```python
from build123d import *

# Parameters (mm, degrees)
BOSS_EXTRUDE1_DEPTH = 1.5
SKETCH3_R           = 7.5
SKETCH3_R_2         = 1.5
SKETCH3_W           = 12
SKETCH3_H           = 23
SKETCH3_W_2         = 5.25
SKETCH3_H_2         = 1.5
CUT_EXTRUDE1_DEPTH  = 66.639165138


with BuildPart() as part:
    # Sketch2 → Boss-Extrude1 (new body)
    with BuildSketch(Plane(origin=(0, 0, 0), x_dir=(1, 0, 0), z_dir=(0, 1, 0))):
        with BuildLine():
            Line((-26.339134382, 42.5), (26.339134382, 42.5))
            ThreePointArc((26.339134382, 42.5), (50, 0), (26.339134382, -42.5))
            Line((26.339134382, -42.5), (-26.339134382, -42.5))
            ThreePointArc((-26.339134382, -42.5), (-50, 0), (-26.339134382, 42.5))
        make_face()
    extrude(amount=BOSS_EXTRUDE1_DEPTH)

    # Sketch3 → Cut-Extrude1 (cut, through all)
    with BuildSketch(Plane(origin=(0, 1.5, 0), x_dir=(1, 0, 0), z_dir=(0, 1, 0))):
        with Locations(Location((0, 0, 0), (0, 0, 270))):
            Circle(SKETCH3_R)
        with Locations(Location((-47, 0, 0), (0, 0, 270))):
            Circle(SKETCH3_R_2)
        with Locations(Location((-33.466401061, 33, 0), (0, 0, 270))):
            Circle(SKETCH3_R_2)
        with Locations(Location((-12.966401061, 33, 0), (0, 0, 270))):
            Circle(SKETCH3_R_2)
        with Locations(Location((-40, 0, 0), (0, 0, 270))):
            Circle(SKETCH3_R_2)
        with Locations(Location((-12.966401061, -33, 0), (0, 0, 90))):
            Circle(SKETCH3_R_2)
        with Locations(Location((-33.466401061, -33, 0), (0, 0, 90))):
            Circle(SKETCH3_R_2)
        with Locations(Location((33.466401061, 33, 0), (0, 0, 90))):
            Circle(SKETCH3_R_2)
        with Locations(Location((12.966401061, 33, 0), (0, 0, 90))):
            Circle(SKETCH3_R_2)
        with Locations(Location((12.966401061, -33, 0), (0, 0, 270))):
            Circle(SKETCH3_R_2)
        with Locations(Location((33.466401061, -33, 0), (0, 0, 270))):
            Circle(SKETCH3_R_2)
        with Locations(Location((40, 0, 0), (0, 0, 90))):
            Circle(SKETCH3_R_2)
        with Locations(Location((47, 0, 0), (0, 0, 90))):
            Circle(SKETCH3_R_2)
        with Locations((-31, -5)):
            Rectangle(SKETCH3_W, SKETCH3_H)
        with Locations((0, -22.5)):
            Rectangle(SKETCH3_W_2, SKETCH3_H_2)
        with Locations((-9.95, 22.5)):
            Rectangle(SKETCH3_W_2, SKETCH3_H_2)
        with Locations((0, 22.5)):
            Rectangle(SKETCH3_W_2, SKETCH3_H_2)
        with Locations((-9.95, -22.5)):
            Rectangle(SKETCH3_W_2, SKETCH3_H_2)
    extrude(amount=-CUT_EXTRUDE1_DEPTH, mode=Mode.SUBTRACT)


solid = part.part
```
Verification items for the finished model (mm, model axes). Coordinates: 2 decimals unless noted, no trailing zeros. Loops run counter-clockwise (first coordinate to the right, second up) from the corner with the lowest first, then second, coordinate; pieces in that order, holes last. Notation, with made-up numbers: (-35, 82.5) -> (3, 82.5) arc R32 cw to (3, 118.5) -> close; hole circle Ø5 at (68, 7.5). An arc over 180 degrees is marked (long way). Answer in a Markdown table with one row per item.
1) Section check B-B (z = 0). Record the cut outline in (x, y).
The answers:
| item | result |
|---|---|
| outline | (-50, 0) -> (-48.5, 0) -> (-48.5, 1.5) -> (-50, 1.5) -> close; (-45.5, 0) -> (-41.5, 0) -> (-41.5, 1.5) -> (-45.5, 1.5) -> close; (-38.5, 0) -> (-37, 0) -> (-37, 1.5) -> (-38.5, 1.5) -> close; (-25, 0) -> (-7.5, 0) -> (-7.5, 1.5) -> (-25, 1.5) -> close; (7.5, 0) -> (38.5, 0) -> (38.5, 1.5) -> (7.5, 1.5) -> close; (41.5, 0) -> (45.5, 0) -> (45.5, 1.5) -> (41.5, 1.5) -> close; (48.5, 0) -> (50, 0) -> (50, 1.5) -> (48.5, 1.5) -> close |
2) Section check D-D (z = 33). Record the cut outline in (x, y).
The answers:
| item | result |
|---|---|
| outline | (-37.56, 0) -> (-34.97, 0) -> (-34.97, 1.5) -> (-37.56, 1.5) -> close; (-31.97, 0) -> (-14.47, 0) -> (-14.47, 1.5) -> (-31.97, 1.5) -> close; (-11.47, 0) -> (11.47, 0) -> (11.47, 1.5) -> (-11.47, 1.5) -> close; (14.47, 0) -> (31.97, 0) -> (31.97, 1.5) -> (14.47, 1.5) -> close; (34.97, 0) -> (37.56, 0) -> (37.56, 1.5) -> (34.97, 1.5) -> close |
3) Draft check along Z on faces 1 (the face through (1, 0, 9)), 2 (the face through (49.995, 0.74, -0.711)), 3 (the face through (12.9, 0.8, -31.5)). Enter one of: released by +Z, released by -Z, zero draft, split by the parting line, or undercut.
The answers:
| item | result |
|---|---|
| face 1 | zero draft |
| face 2 | split by the parting line |
| face 3 | undercut |
4) Scan lines: line 1 along X through (y, z) = (0.3, -33); line 2 along Z through (x, y) = (12, 1.05); line 3 along Z through (x, y) = (-1, 0.4). Record each from-to range of solid material in increasing order. Write a range as from..to.
The answers:
| item | result |
|---|---|
| line 1 | x = -37.56..-34.97, -31.97..-14.47, -11.47..11.47, 14.47..31.97, 34.97..37.56 |
| line 2 | z = -42.5..-34.15, -31.85..31.85, 34.15..42.5 |
| line 3 | z = -42.5..-23.25, -21.75..-7.43, 7.43..21.75, 23.25..42.5 |
5) Section check A-A (x = 0). Record the cut outline in (y, z).
The answers:
| item | result |
|---|---|
| outline | (0, -42.5) -> (1.5, -42.5) -> (1.5, -23.25) -> (0, -23.25) -> close; (0, -21.75) -> (1.5, -21.75) -> (1.5, -7.5) -> (0, -7.5) -> close; (0, 7.5) -> (1.5, 7.5) -> (1.5, 21.75) -> (0, 21.75) -> close; (0, 23.25) -> (1.5, 23.25) -> (1.5, 42.5) -> (0, 42.5) -> close |
6) Section check C-C (x = -40). Record the cut outline in (y, z).
The answers:
| item | result |
|---|---|
| outline | (0, -30) -> (1.5, -30) -> (1.5, -1.5) -> (0, -1.5) -> close; (0, 1.5) -> (1.5, 1.5) -> (1.5, 30) -> (0, 30) -> close |
7) Depth check by flat-ended pin: P1, Ø0.8, axis at x = -30.5, y = 1, coming from the -Z side. Enter the tip coordinate at first touch or a pass-through.
The answers:
| item | result |
|---|---|
| P1 | stops at z = -39.92 |
